CAD build for the part. Positions are in the model's coordinates, mm. Face numbers are marked on the shaded views. A direction names the side the tool comes from. Coordinates: 2 decimals unless noted, no trailing zeros. Order: outer loops, then holes, each group sorted by start corner. A loop starts at its lowest first (then second) coordinate and runs counter-clockwise, first axis right, second up.
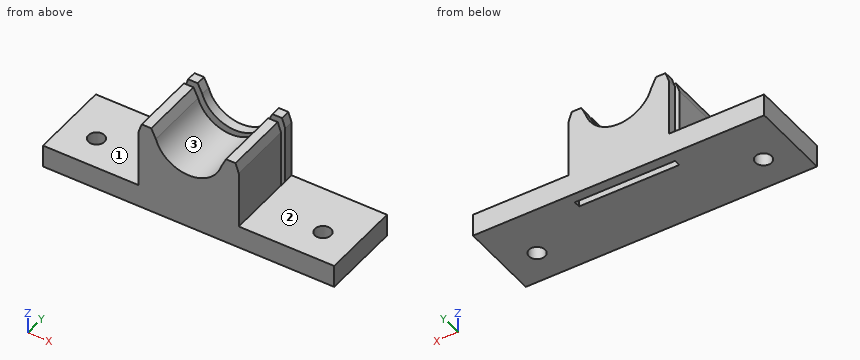
Autodesk Inventor part; units mm, degrees
ref_plane "YZ Plane" through (0, 0, 0) normal (1, 0, 0) x (0, 1, 0)
ref_plane "XZ Plane" through (0, 0, 0) normal (0, 1, 0) x (-1, 0, 0)
ref_plane "XY Plane" through (0, 0, 0) normal (0, 0, 1) x (1, 0, 0)
sketch "Sketch1" plane through (0, 0, 0) normal (0, 0, 1) x (1, 0, 0)
  line L0 (-45, 10) -> (45, 10)
  line L1 (45, 10) -> (45, -10)
  line L2 (45, -10) -> (-45, -10)
  line L3 (-45, -10) -> (-45, 10)
  point P0 (0, 0)
  point P1 (0, 10)
  point P2 (-45, 0)
  dimension "d0" = 20
  dimension "d1" = 90
extrude "Extrusion1" add sketch "Sketch1" along normal blind 27.75
sketch "Sketch3" plane through (-45, 10, 0) normal (0, 1, 0) x (1, 0, 0)
  line L0 (90, 0) -> (90, -27.75)
  line L1 (90, -27.75) -> (0, -27.75)
  line L2 (90, -27.75) -> (60.5, -27.75)
  line L3 (60.5, -27.75) -> (60.5, -7)
  line L4 (60.5, -7) -> (90, -7)
  line L5 (90, -7) -> (90, -27.75)
  line L6 (83, -7) -> (95, -7)
  line L7 (90, 0) -> (0, 0)
  point P0 (45, 0)
  point P1 (60.5, -27.75)
  dimension "d8" = 20.75
  dimension "d20" = 15.5
  dimension "d40" = 7
extrude "Extrusion2" cut sketch "Sketch3" against normal through all
mirror "Mirror1" about plane through (0, 0, 0) normal (1, 0, 0) of "Extrusion2"
sketch "Sketch4" plane through (-45, 10, 0) normal (0, 1, 0) x (1, 0, 0)
  circle A0 centre (45, -27.75) radius 10.55
  line L0 (90, 0) -> (0, 0)
  line L1 (60.5, -27.75) -> (29.5, -27.75)
  point P0 (45, 0)
  point P1 (45, 0)
  dimension "d32" = 21.1
  dimension "d39" = 0
extrude "Extrusion3" cut sketch "Sketch4" against normal through all
chamfer "Chamfer1" distance 1 distance2 3 1 edges at (-15.5, 0, 27.75) measured on face at (-12.2, -3.3333, 27.75)
chamfer "Chamfer2" distance 1 distance2 3 1 edges at (15.5, 0, 27.75) measured on face at (12.2, 3.3333, 27.75)
sketch "Sketch5" plane through (0, 0, 0) normal (0, 0, -1) x (-1, 0, 0)
  line L0 (45, -10) -> (-45, -10)
  line L1 (0, 23.0048) -> (0, -23.0048) construction
  point P0 (0, 0)
  point P1 (-35, 0)
  point P2 (35, 0)
  point P3 (0, 0)
  dimension "d23" = 70
hole "Hole1" at (35, 0, 0) at (-35, 0, 0) direction (0, 0, 1) diameter 5 end through all
chamfer "Chamfer3" distance 1 distance2 3 2 edges at (10.55, 0, 27.75) (-10.55, 0, 27.75) measured on face at (13.1833, -3.3333, 27.75) measured on face at (-13.1833, -3.3333, 27.75)
chamfer_without_effect "Chamfer4"
sketch "Sketch6" plane through (-45, 10, 0) normal (0, 1, 0) x (1, 0, 0)
  line L0 (56.55, -27.75) -> (55.1235, -24.7805)
  line L1 (59.5, -27.75) -> (56.55, -27.75)
  line L2 (60.5, -24.75) -> (59.5, -27.75)
  line L3 (60.5, -24.75) -> (60.5, -7)
  line L4 (60.5, -7) -> (90, -7)
  line L5 (90, 0) -> (90, -7)
  line L6 (90, 0) -> (0, 0)
  line L7 (0, 0) -> (0, -7)
  line L8 (0, -7) -> (29.5, -7)
  line L9 (29.5, -7) -> (29.5, -24.75)
  line L10 (30.5, -27.75) -> (29.5, -24.75)
  line L11 (33.45, -27.75) -> (30.5, -27.75)
  line L12 (34.8765, -24.7805) -> (33.45, -27.75)
  arc A0 (55.1235, -24.7805) -> (34.8765, -24.7805) centre (45, -27.75) ccw
  point P0 (45, 0)
extrude "Extrusion4" add sketch "Sketch6" along normal blind 5
sketch "Sketch7" plane through (-45, -10, 7) normal (0, 0, 1) x (1, 0, 0)
  line L0 (13, 20) -> (27.9, 20)
  line L1 (29.5, 22) -> (60.5, 22)
  line L2 (60.5, 22) -> (60.5, 20)
  line L3 (60.5, 20) -> (29.5, 20)
  line L4 (29.5, 20) -> (29.5, 22)
  line L5 (60.5, 25) -> (60.5, 0)
  line L6 (29.5, 25) -> (29.5, 0)
  point P0 (45, 10)
  dimension "d43" = 2
extrude "Extrusion5" cut sketch "Sketch7" along normal through all both and the other way through all
properties part number "0008-10-057  Fixare seringa 20 Ml" material "ABS Plastic"
1) Which spindle directions (+Z, -Z, +X, -X, +Y, -Y) get a long thin tool onto all of the face, cutting with end or side? Do the marked faces 1, 2 and 3. Say none if no direction does.
2) Drill centre lines: probe 1 along X at (y, z) = (0, 5.25); probe 2 along Y at (x, z) = (-35, 5.5); probe 3 along Z at (x, y) = (-38, 14). Where is each one in solid material? Low to high.
3) Pin check, flat tips, straight feed: P1, Ø4, axis at x = -35, y = 0, coming from the -Z side; P2, Ø0.9, axis at y = 13, z = 15.5, coming from the +X side; P3, Ø5, axis at x = -22.5, y = 12, coming from the +Z side; P4, Ø5.5, axis at y = 2, z = 17.5, coming from the -X side. Stop position of each tip, or through.
4) Slice it at C-C (x = 35). List the corners of the cut face in (y, z).
5) Slice it at A-A (y = 0). List the corners of the cut face in (x, z).
6) Slice it at D-D (z = 10). List the corners of the cut face in (x, y).
7) Slice it at B-B (z = 2). List the corners of the cut face in (x, y).
Worked out:
1. face 1: +Z, -X, +Y, -Y
1. face 2: +Z, +X, +Y, -Y
1. face 3: +Z, +Y, -Y
2. probe 1: x = -45 to -37.5, -32.5 to 32.5, 37.5 to 45
2. probe 2: y = -10 to -2.5, 2.5 to 15
2. probe 3: z = 0 to 7
3. P1: passes through
3. P2: stops at x = 15.5
3. P3: stops at z = 7
3. P4: stops at x = -15.5
4. outline: (-10, 0) - (-2.5, 0) - (-2.5, 7) - (-10, 7) - close; (2.5, 0) - (15, 0) - (15, 7) - (2.5, 7) - close
5. outline: (-45, 0) - (-37.5, 0) - (-37.5, 7) - (-45, 7) - close; (-32.5, 0) - (32.5, 0) - (32.5, 7) - (15.5, 7) - (15.5, 24.75) - (14.5, 27.75) - (11.55, 27.75) - (10.12, 24.78) arc R10.55 cw to (-10.12, 24.78) - (-11.55, 27.75) - (-14.5, 27.75) - (-15.5, 24.75) - (-15.5, 7) - (-32.5, 7) - close; (37.5, 0) - (45, 0) - (45, 7) - (37.5, 7) - close
6. outline: (-15.5, -10) - (15.5, -10) - (15.5, 10) - (-15.5, 10) - close; (-15.5, 12) - (15.5, 12) - (15.5, 15) - (-15.5, 15) - close
7. outline: (-45, -10) - (45, -10) - (45, 15) - (-45, 15) - close; hole circle Ø5 at (-35, 0); hole (-15.5, 10) - (15.5, 10) - (15.5, 12) - (-15.5, 12) - close; hole circle Ø5 at (35, 0)
